Work out the finished part from the listing and answer in its coordinate system (mm). A direction names the side the tool comes from. Coordinates: 2 decimals unless noted, no trailing zeros. Write each loop counter-clockwise with the first axis right and the second up, starting at its lowest first coordinate (ties: lowest second). Pieces come first, ordered by that corner, then holes. Notation, with made-up numbers: (34.25, 24.5) - (81.25, 24.5) arc R15 ccw to (81.25, 30.5) - close; hole circle Ø10 at (84, 17.5). An arc over 180 degrees is marked (long way). One line per item, written item: value.
Autodesk Inventor part; units mm, degrees
ref_plane "YZ Plane" through (0, 0, 0) normal (1, 0, 0) x (0, 1, 0)
ref_plane "XZ Plane" through (0, 0, 0) normal (0, 1, 0) x (-1, 0, 0)
ref_plane "XY Plane" through (0, 0, 0) normal (0, 0, 1) x (1, 0, 0)
sketch "Sketch1" plane through (0, 0, 0) normal (0, 0, 1) x (1, 0, 0)
  line L0 (-4, 9.5) -> (4, 9.5)
  line L1 (4, 9.5) -> (4, -9.5)
  line L2 (4, -9.5) -> (-4, -9.5)
  line L3 (-4, -9.5) -> (-4, 9.5)
  line L4 (-4, 9.5) -> (4, -9.5) construction
  line L5 (4, 9.5) -> (-4, -9.5) construction
  line L6 (4, 9.5) -> (8, 9.5)
  line L7 (8, 9.5) -> (8, 4.5)
  line L8 (8, 4.5) -> (4, 4.5)
  line L9 (4, 4.5) -> (4, 9.5)
  line L10 (8, -0.5) -> (4, -0.5)
  line L11 (8, 4.5) -> (8, -0.5)
  line L12 (8, -5.5) -> (4, -5.5)
  line L13 (8, -0.5) -> (8, -5.5)
  line L14 (2, 14.112) -> (2, 5.4586)
  line L15 (0, 9.5) -> (0, -9.5)
  line L16 (0, 9.5) -> (-4, 9.5)
  line L17 (-4, 9.5) -> (-4, 4.5)
  line L18 (-4, 4.5) -> (0, 4.5)
  line L19 (-4, -0.5) -> (0, -0.5)
  line L20 (-4, 4.5) -> (-4, -0.5)
  line L21 (-4, -0.5) -> (-4, -9.5)
  line L22 (-4, -5.5) -> (0, -5.5)
  point P0 (0, 0)
  point P1 (0, 4.5)
  point P2 (-4, 4.5)
  point P3 (-4, -0.5)
  point P4 (4, -7)
  point P5 (8, -0.5)
  point P6 (0, 9.5)
  point P7 (8, 4.5)
  point P8 (4, -5.5)
  point P9 (0, -5.5)
  point P10 (-4, -5.5)
  dimension "d0" = 8
  dimension "d1" = 19
  dimension "d2" = 4
  dimension "d3" = 5
  dimension "d6" = 5
  dimension "d11" = 12
  dimension "d12" = 6
extrude "Extrusion1" add sketch "Sketch1" along normal blind 4 contours L0 L1 L2 L15 | L18 L15 L19 L3 | L6 L7 L8 L1 | L22 L15 L2 L3 | L10 L13 L12 L1
sketch "Sketch2" plane through (0, 0, 4) normal (0, 0, 1) x (1, 0, 0)
  line L0 (0, -5.5) -> (-4, -5.5)
  line L1 (-4, -5.5) -> (-4, -9.5)
  line L2 (-4, -9.5) -> (4, -9.5)
  line L3 (4, -9.5) -> (4, -5.5)
  line L4 (4, -5.5) -> (8, -5.5)
  line L5 (8, -5.5) -> (8, -0.5)
  line L6 (8, -0.5) -> (4, -0.5)
  line L7 (4, -0.5) -> (4, 4.5)
  line L8 (4, 4.5) -> (8, 4.5)
  line L9 (8, 4.5) -> (8, 9.5)
  line L10 (8, 9.5) -> (0, 9.5)
  line L11 (0, 9.5) -> (0, 4.5)
  line L12 (0, 4.5) -> (-4, 4.5)
  line L13 (-4, 4.5) -> (-4, -0.5)
  line L14 (-4, -0.5) -> (0, -0.5)
  line L15 (0, -0.5) -> (0, -5.5)
  point P0 (0, 0)
equation "\"d1\" = height + e"
equation "\"d2\" = e"
equation "\"d3\" = 0.333333 * height"
equation "\"d6\" = d3"
equation "\"d12\" = 0.5 * d11"
equation "\"d13\" = e"
equation "\"e\" = 4"
equation "\"height\" = 15"
properties part number "wall2" material "MDF Medium Density Fiberboard"
Item 1: Given pin 1 (2 mm diameter, centred on x = 6, z = 1.5, fed in from -Y); pin 2 (4 mm diameter, centred on x = 4, y = 1.5, fed in from -Z); pin 3 (2 mm diameter, centred on y = -3, z = 1.5, fed in from -X); pin 4 (2 mm diameter, centred on x = -2, z = 3, fed in from +Y), each flat-ended and moving along its own axis, determine where each tip first touches the part or whether it passes through.
Evaluation:
pin 1: stops at y = -5.5
pin 2: stops at z = 0
pin 3: stops at x = 0
pin 4: stops at y = 4.5
Item 2: Section B-B, the plane z = 2.95 is taken. Determine the outline of the cut face in (x, y), then the cut area to 3 significant figures.
Evaluation:
outline: (-4, -9.5) - (4, -9.5) - (4, -5.5) - (8, -5.5) - (8, -0.5) - (4, -0.5) - (4, 4.5) - (8, 4.5) - (8, 9.5) - (0, 9.5) - (0, 4.5) - (-4, 4.5) - (-4, -0.5) - (0, -0.5) - (0, -5.5) - (-4, -5.5) - close
area: 152 mm2
Item 3: Section C-C, the plane y = 1 is taken. Determine the outline of the cut face in (x, z).
Evaluation:
outline: (-4, 0) - (4, 0) - (4, 4) - (-4, 4) - close
Item 4: Section A-A, the plane x = 6.5 is taken. Determine the outline of the cut face in (y, z).
Evaluation:
outline: (-5.5, 0) - (-0.5, 0) - (-0.5, 4) - (-5.5, 4) - close; (4.5, 0) - (9.5, 0) - (9.5, 4) - (4.5, 4) - close
Item 5: Determine the mould class of faces 1 (the face through (6, -5.5, 2)), 2 (the face through (4, 2, 2)), 3 (the face through (4, 9.5, 2)), 4 (the face through (6, 4.5, 2)) for opening direction Y: +Y half, -Y half, draft (parallel to the pull), parting line (faces both ways), or undercut.
Evaluation:
face 1: -Y half
face 2: undercut
face 3: +Y half
face 4: undercut
Item 6: Consider probe 1 along Y at (x, z) = (6.75, 1.15); probe 2 along Y at (x, z) = (-2.25, 3.3); probe 3 along X at (y, z) = (7.5, 3.35). Determine where each line is inside the solid, lowest interval first.
Evaluation:
probe 1: y = -5.5 to -0.5, 4.5 to 9.5
probe 2: y = -9.5 to -5.5, -0.5 to 4.5
probe 3: x = 0 to 8
Item 7: Which of the six approach directions +Z, -Z, +X, -X, +Y, -Y give full straight-line access (tool end or side, diameter ignored) to faces 5 (the face through (4, -7, 2)), 6 (the face through (0, 7, 2)), 7 (the face through (0, -3, 2))?
Evaluation:
face 5: +Z, -Z, +X, -Y
face 6: +Z, -Z, -X, +Y
face 7: +Z, -Z, -X
